Autodesk Inventor part; units mm, degrees
ref_plane "YZ Plane" through (0, 0, 0) normal (1, 0, 0) x (0, 1, 0)
ref_plane "XZ Plane" through (0, 0, 0) normal (0, 1, 0) x (-1, 0, 0)
ref_plane "XY Plane" through (0, 0, 0) normal (0, 0, 1) x (1, 0, 0)
sketch "Sketch1" plane through (0, 0, 0) normal (0, 1, 0) x (-1, 0, 0)
  line L0 (0, 0) -> (0, 101.6)
  line L1 (0, 101.6) -> (-12.7, 101.6)
  line L2 (0, 0) -> (-44.45, 0)
  line L3 (-12.7, 101.6) -> (-50.3351, 8.735)
  arc A0 (-50.3351, 8.735) -> (-44.45, 0) centre (-44.45, 6.35) ccw
  line L4 (-50.8, 8.1746) -> (-50.8, -12.3493) construction
  circle A1 centre (-22.225, 22.225) radius 12.7
  point P0 (-53.8751, 0)
  dimension "d0" = 101.6
  dimension "d1" = 12.7
  dimension "d4" = 6.35
  dimension "d5" = 50.8
  dimension "d6" = 25.4
  dimension "d7" = 22.225
  dimension "d8" = 22.225
extrude "Extrusion1" add sketch "Sketch1" along normal blind 4.7625
ref_plane "WP Lug" through (0, 2.3813, 0) normal (0, 1, 0) x (1, 0, 0)
properties part number "Liftinglug"
For this review, take the finished solid that the model builds, in its own axes (mm). Round coordinates to 2 decimals unless told otherwise and drop trailing zeros. Loops run counter-clockwise (first coordinate to the right, second up) from the corner with the lowest first, then second, coordinate; pieces in that order, holes last. Notation, with made-up numbers: (40.25, 6) - (65.25, 6) arc R28 ccw to (65.25, 38) - close; hole circle Ø5 at (14.5, 13.25). An arc over 180 degrees is marked (long way). Put each result on its own line as item: value. Start each with the question number.
1. Mouldability with a two-part tool opening along Z and no side actions: class faces 1 (the cylindrical face through (23.878, 2.348, 9.633)), 2 (the flat face through (20, 4.762, 40)), 3 (the flat face through (6, 2, 101.6)), 4 (the flat face through (22, 2, 0)) as +Z half, -Z half, draft (parallel to the pull), parting line (faces both ways), or undercut.
2. Consider section B-B on x = 16. State the section outline as (y, z) points, plus the area to 3 significant figures.
3. Consider section A-A on z = 28. State the section outline as (x, y) points, plus the area to 3 significant figures.
4. Consider section D-D on x = 42.5. State the section outline as (y, z) points.
5. Consider section C-C on y = 3.8. State the section outline as (x, z) points (3 decimals), plus the area to 3 significant figures.
6. Insertion check: P1, Ø1.5, axis at y = 2, z = 18.5, coming from the -X side. The pin has a flat end and moves straight along its axis. Give the tip position at first contact, or say it passes through.
7. For probe 1 along Z at (x, y) = (13, 2.7); probe 2 along Z at (x, y) = (17.5, 1.4); probe 3 along X at (y, z) = (4, 29), list the stretches that pass through material, from the lowest coordinate up. Write a range as [from, to].
Result sheet:
1. face 1: undercut
1. face 2: draft
1. face 3: +Z half
1. face 4: -Z half
2. outline: (0, 0) - (4.76, 0) - (4.76, 11.16) - (0, 11.16) - close; (0, 33.29) - (4.76, 33.29) - (4.76, 93.46) - (0, 93.46) - close
2. area: 340 mm^2
3. outline: (0, 0) - (10.91, 0) - (10.91, 4.76) - (0, 4.76) - close; (33.54, 0) - (42.53, 0) - (42.53, 4.76) - (33.54, 4.76) - close
3. area: 94.8 mm^2
4. outline: (0, 0) - (4.76, 0) - (4.76, 28.07) - (0, 28.07) - close
5. outline: (0, 0) - (44.45, 0) arc R6.35 ccw to (50.335, 8.735) - (12.7, 101.6) - (0, 101.6) - close; hole circle Ø25.4 at (22.225, 22.225)
5. area: 2,850 mm^2
6. P1: x = 0
7. probe 1: [0, 13.5], [30.95, 100.86]
7. probe 2: [0, 10.44], [34.01, 89.76]
7. probe 3: [0, 11.48], [32.97, 42.12]
